```python
from build123d import *

# Parameters (mm, degrees)
F0_W     = 50.8
F0_H     = 12.7
F1_DEPTH = 31.75
F2_W     = 50.8
F2_H     = 15.875
F3_DEPTH = 19.05
F5_DEPTH = 25.4
F6_W     = 12.7
F6_H     = 15.875
F7_DEPTH = 19.05
F9_DEPTH = 31.751


with BuildPart() as f1:
    # F0 (on Front) → F1 (new body)
    with BuildSketch(Plane.XZ):
        with Locations((25.4, -6.35)):
            Rectangle(F0_W, F0_H)
    extrude(amount=F1_DEPTH)

    # F2 (on face) → F3 (join)
    with BuildSketch(Plane.XY):
        with Locations((25.4, -7.9375)):
            Rectangle(F2_W, F2_H)
    extrude(amount=F3_DEPTH)

    # F4 (on face) → F5 (cut)
    with BuildSketch(Plane.XZ.offset(15.875)):
        Polygon((50.8, 0), (50.8, 19.05), (38.1, 19.05), align=None)
    extrude(amount=-F5_DEPTH, mode=Mode.SUBTRACT)

    # F6 (on face) → F7 (join)
    with BuildSketch(Plane.XY):
        with Locations((25.4, -23.8125)):
            Rectangle(F6_W, F6_H)
    extrude(amount=F7_DEPTH)

    # F8 (on face) → F9 (cut, through all)
    with BuildSketch(Plane.YZ.offset(31.75)):
        Polygon((-31.75, 0), (-15.875, 19.05), (-31.75, 19.05), align=None)
    extrude(amount=-F9_DEPTH, mode=Mode.SUBTRACT)


solid = f1.part
```
The model under review builds one solid part; all positions refer to its coordinate system, in mm. A direction names the side the tool comes from. Round coordinates to 2 decimals unless told otherwise and drop trailing zeros. Loops run counter-clockwise (first coordinate to the right, second up) from the corner with the lowest first, then second, coordinate; pieces in that order, holes last. Notation, with made-up numbers: (3.25, 79) - (32.25, 79) arc R11 cw to (32.25, 99) - close; hole circle Ø9 at (40, 59). An arc over 180 degrees is marked (long way). Use a Markdown table: item, result. Add a question column.
Q1. Add section D-D (y = -8.5). State the section outline as (x, z) points, plus the area to 3 significant figures.
Q2. Add section A-A (y = -28). State the section outline as (x, z) points, plus the area to 3 significant figures.
Q3. For probe 1 along Z at (x, y) = (17, -25.5); probe 2 along X at (y, z) = (-16, 12); probe 3 along Y at (x, z) = (5, 10.5) (3 decimals), list the stretches that pass through material, from the lowest coordinate up.
Q4. Add section B-B (x = 15). State the section outline as (y, z) points (3 decimals).
Q5. Add section C-C (z = 1). State the section outline as (x, y) points (3 decimals), plus the area to 3 significant figures.
Q6. Insertion check: pin 1 Ø9.5 at (x, z) = (11, 12) entering from -Y (3 decimals); pin 2 Ø6 at (y, z) = (-25, 12) entering from +X; pin 3 Ø17.5 at (y, z) = (-22, 11.5) entering from +X. Each pin has a flat end and moves straight along its axis. Give the tip position at first contact, or say it passes through.
Q7. Machinability: for faces 1 (the face through (44.36, -8.05, 9.66)), 2 (the face through (9, -15.875, 9)), 3 (the face through (41, -24, 0)), which of the approach directions +Z, -Z, +X, -X, +Y, -Y give a long, thin tool a straight path to every point of the face, cutting with its end or side? Answer none if there is none.
Worked answers:
| question | item | result |
|---|---|---|
| 1 | outline | (0, -12.7) - (50.8, -12.7) - (50.8, 0) - (38.1, 19.05) - (0, 19.05) - close |
| 1 | area | 1,490 mm² |
| 2 | outline | (0, -12.7) - (50.8, -12.7) - (50.8, 0) - (31.75, 0) - (31.75, 4.5) - (19.05, 4.5) - (19.05, 0) - (0, 0) - close |
| 2 | area | 702 mm² |
| 3 | probe 1 | -12.7 to 0 |
| 3 | probe 2 | 19.05 to 31.75 |
| 3 | probe 3 | -15.875 to 0 |
| 4 | outline | (-31.75, -12.7) - (0, -12.7) - (0, 19.05) - (-15.875, 19.05) - (-15.875, 0) - (-31.75, 0) - close |
| 5 | outline | (0, -15.875) - (19.05, -15.875) - (19.05, -30.917) - (31.75, -30.917) - (31.75, -15.875) - (50.133, -15.875) - (50.133, 0) - (0, 0) - close |
| 5 | area | 987 mm² |
| 6 | pin 1 | y = -15.875 |
| 6 | pin 2 | x = 31.75 |
| 6 | pin 3 | x = 47.3 |
| 7 | face 1 | +Z, +X, +Y, -Y |
| 7 | face 2 | +Z, -X, -Y |
| 7 | face 3 | +Z, +X, -Y |
